Build history of the part. All positions in model axes, mm. A direction names the side the tool comes from. Round coordinates to 2 decimals unless told otherwise and drop trailing zeros. Order: outer loops, then holes, each group sorted by start corner. A loop starts at its lowest first (then second) coordinate and runs counter-clockwise, first axis right, second up. Notation, with made-up numbers: (-22.5, -38.5) -> (33.5, -38.5) arc R33 cw to (33.5, 0.5) -> close; hole circle Ø2 at (15, 62). An arc over 180 degrees is marked (long way). Answer as CSV lines item,"result". Start each with the question number.
```python
from build123d import *
from build123d.topology import SkipClean

# Parameters (mm, degrees)
BOSS_EXTRUDE1_DEPTH = 10
SKETCH2_R           = 30
BOSS_EXTRUDE2_DEPTH = 20
SKETCH3_W           = 165
SKETCH3_H           = 50
BOSS_EXTRUDE3_DEPTH = 10


with BuildPart() as part:
    # Sketch1 → Boss-Extrude1 (new body)
    with BuildSketch(Plane.XY):
        with BuildLine():
            Line((-165, 30), (-215, 30))
            ThreePointArc((-215, 30), (-245, 0), (-215, -30))
            Line((-215, -30), (-165, -30))
            Line((-165, -30), (-165, -55.06097561))
            Line((-165, -55.06097561), (-100, -55.06097561))
            Line((-100, -55.06097561), (-100, -30))
            Line((-100, -30), (-50, -30))
            Line((-50, -30), (-50, 30))
            Line((-50, 30), (-100, 30))
            Line((-100, 30), (-100, 55.06097561))
            Line((-100, 55.06097561), (-165, 55.06097561))
            Line((-165, 55.06097561), (-165, 30))
        make_face()
    boss_extrude1 = extrude(amount=BOSS_EXTRUDE1_DEPTH)

    # Sketch2 → Boss-Extrude2 (add)
    with SkipClean():  # the faces are left unmerged after this step: merging them gives an invalid solid
        with BuildSketch(Plane.XY.offset(10)):
            with Locations(Location((-215, 0, 0), (0, 0, 270))):
                Circle(SKETCH2_R)
        boss_extrude2 = extrude(amount=BOSS_EXTRUDE2_DEPTH)

    # Sketch3 → Boss-Extrude3 (add)
    with BuildSketch(Plane.XZ.offset(30)):
        with Locations((-132.5, -15)):
            Rectangle(SKETCH3_W, SKETCH3_H)
    extrude(amount=-BOSS_EXTRUDE3_DEPTH)

    # Mirror1: Boss-Extrude1, Boss-Extrude2 across plane
    with SkipClean():  # the faces are left unmerged after this step: merging them gives an invalid solid
        add(boss_extrude1.mirror(Plane.XY.offset(-15)))
        add(boss_extrude2.mirror(Plane.XY.offset(-15)))
    add(part.part.scale(1), mode=Mode.REPLACE)  # the faces are merged on a copy


solid = part.part
```
Q1. Slice it at B-B, the plane x = -141.5. Write the cut outline in (y, z), plus the area to 3 significant figures.
Q2. Slice it at D-D, the plane z = 15. Write the cut outline in (x, y), plus the area to 3 significant figures.
Q3. Slice it at A-A, the plane y = -41. Write the cut outline in (x, z), plus the area to 3 significant figures.
Q4. Probe L1, parallel to Z at x = -131, y = 18; L2, parallel to Z at x = -204.5, y = -1; L3, parallel to Y at x = -61, z = 6. List the from-to ranges inside material, lowest first.
Q5. Which spindle directions (+Z, -Z, +X, -X, +Y, -Y) get a long thin tool onto all of the face, cutting with end or side? Do faces 5 (the face through (-165, 43, 5)), 6 (the face through (-134, -20, -15)), 7 (the face through (-75, 30, -35)). Say none if no direction does.
Q6. Flat gauge pins, fed straight in: pin 1 Ø3 at (y, z) = (-46, 3.5) entering from +X; pin 2 Ø8 at (y, z) = (34, -29.5) entering from -X; pin 3 Ø6 at (x, y) = (-90, -8) entering from -Z; pin 4 Ø1.5 at (y, z) = (-18.5, -23) entering from -X (3 decimals). Where does each tip first touch, or does it go through?
Q7. Two-plate mould, pull along Z, no slides. Class faces 1 (the face through (-100, 42, 5)), 2 (the face through (-215, 0, -60)), 3 (the face through (-134, -30, -15)), 4 (the face through (-115, 1, 10)): +Z half, -Z half, draft (parallel to the pull), parting line (faces both ways), or undercut.
Solutions:
1,outline,"(-55.06, -40) -> (55.06, -40) -> (55.06, -30) -> (-20, -30) -> (-20, 0) -> (55.06, 0) -> (55.06, 10) -> (-55.06, 10) -> (-55.06, 0) -> (-30, 0) -> (-30, -30) -> (-55.06, -30) -> close"
1,area,"2,500 mm2"
2,outline,"circle Ø60 at (-215, 0)"
2,area,"2,830 mm2"
3,outline,"(-165, -40) -> (-100, -40) -> (-100, -30) -> (-165, -30) -> close; (-165, 0) -> (-100, 0) -> (-100, 10) -> (-165, 10) -> close"
3,area,"1,300 mm2"
4,L1,"z = -40 to -30, 0 to 10"
4,L2,"z = -60 to -30, 0 to 30"
4,L3,"y = -30 to 30"
5,face 5,"+Z, -Z, -X, +Y"
5,face 6,"+X, -X, +Y"
5,face 7,"+Z, -Z, +X, +Y"
6,pin 1,"stops at x = -100"
6,pin 2,"stops at x = -165"
6,pin 3,"stops at z = -40"
6,pin 4,"passes through"
7,face 1,"draft"
7,face 2,"-Z half"
7,face 3,"undercut"
7,face 4,"+Z half"
